For this review, take the finished solid that the model builds, in its own axes (mm). A direction names the side the tool comes from. Give positions to 0.01 mm unless a question says otherwise; leave off trailing zeros. Loops run counter-clockwise (first coordinate to the right, second up) from the corner with the lowest first, then second, coordinate; pieces in that order, holes last. Notation, with made-up numbers: (73, 65.25) - (91, 65.25) arc R33 ccw to (91, 99.25) - close; hole circle Ø6 at (88, -34.75). An arc over 180 degrees is marked (long way). Answer in a Markdown table with one row per item.
```python
from build123d import *

# Parameters (mm, degrees)
F0_W     = 136.525
F0_H     = 241.3
F1_DEPTH = 25.4
F3_DEPTH = 25.4


with BuildPart() as f1:
    # F0 (on Front) → F1 (new body)
    with BuildSketch(Plane.XZ):
        Rectangle(F0_W, F0_H)
    extrude(amount=F1_DEPTH)

    # F2 (on face) → F3 (join)
    with BuildSketch(Plane.XZ.offset(25.4)):
        with BuildLine():
            ThreePointArc((77.6254340957, 53.8129340957), (71.9080698474, 61.2266782869), (68.2625, 69.85))
            Line((68.2625, 69.85), (68.2625, -6.35))
            ThreePointArc((68.2625, -6.35), (71.9080698474, 2.2733217131), (77.6254340957, 9.6870659043))
            ThreePointArc((77.6254340957, 9.6870659043), (82.7346936877, 13.9409024845), (88.5302033496, 17.1984670639))
            ThreePointArc((88.5302033496, 17.1984670639), (92.3418278085, 24.0349565831), (93.6625, 31.75))
            ThreePointArc((93.6625, 31.75), (92.3418278085, 39.4650434169), (88.5302033496, 46.3015329361))
            ThreePointArc((88.5302033496, 46.3015329361), (82.7346936877, 49.5590975155), (77.6254340957, 53.8129340957))
        make_face()
        with BuildLine():
            ThreePointArc((88.5302033496, 46.3015329361), (83.6252121519, 50.8519186766), (77.6254340957, 53.8129340957))
            ThreePointArc((77.6254340957, 53.8129340957), (82.7346936877, 49.5590975155), (88.5302033496, 46.3015329361))
        make_face()
        with BuildLine():
            ThreePointArc((88.5302033496, 17.1984670639), (82.7346936877, 13.9409024845), (77.6254340957, 9.6870659043))
            ThreePointArc((77.6254340957, 9.6870659043), (83.6252121519, 12.6480813234), (88.5302033496, 17.1984670639))
        make_face()
    extrude(amount=-F3_DEPTH)

    # F4: F1 across plane


with BuildPart() as f1_1:
    add(f1.part)
    add(f1.part.mirror(Plane.YZ))


solid = f1_1.part
```
1. Wall thickness on line 1 (X direction, y = -1.5, z = 70); line 2 (X direction, y = -7.5, z = 33); line 3 (Z direction, x = 71.5, y = -16.75): over which ranges is each line inside the solid? List them lowest first. Write a range as [from, to].
Values:
| item | result |
|---|---|
| line 1 | x = [-68.26, 68.26] |
| line 2 | x = [-93.63, 93.63] |
| line 3 | z = [1.56, 61.94] |
2. Clearance check with flat-ended pins moving along their axes: pin 1 (4 mm diameter, centred on y = -18.5, z = -6, fed in from +X); pin 2 (12.5 mm diameter, centred on y = -18, z = -74.5, fed in from +X); pin 3 (12.5 mm diameter, centred on y = -15, z = -78, fed in from -X). State where each tip first meets the part, or that it passes through.
Values:
| item | result |
|---|---|
| pin 1 | stops at x = 69 |
| pin 2 | stops at x = 68.26 |
| pin 3 | stops at x = -68.26 |
3. For faces 1 (the face through (68.262, -13, 95)), 2 (the face through (-68.262, -13, 95)), 3 (the face through (-68.262, -13, -64)), list the 3-axis set-ups (+Z, -Z, +X, -X, +Y, -Y) from which the entire face can be reached by the end or side of a thin tool; tool diameter is ignored.
Values:
| item | result |
|---|---|
| face 1 | +Z, +X, +Y, -Y |
| face 2 | +Z, -X, +Y, -Y |
| face 3 | -Z, -X, +Y, -Y |
4. We need section A-A, the plane y = -7.75. Give the boundary of the cut face in (x, z), and give its area (3 significant figures).
Values:
| item | result |
|---|---|
| outline | (-77.63, 9.69) arc R36.54 cw to (-68.26, -6.35) - (-68.26, -120.65) - (68.26, -120.65) - (68.26, -6.35) arc R36.54 cw to (77.63, 9.69) arc R23.2 ccw to (77.63, 53.81) arc R36.54 cw to (68.26, 69.85) - (68.26, 120.65) - (-68.26, 120.65) - (-68.26, 69.85) arc R36.54 cw to (-77.63, 53.81) arc R23.2 ccw to start |
| area | 35,000 mm^2 |
5. We need section B-B, the plane z = 94. Give the boundary of the cut face in (x, y), and give its area (3 significant figures).
Values:
| item | result |
|---|---|
| outline | (-68.26, -25.4) - (68.26, -25.4) - (68.26, 0) - (-68.26, 0) - close |
| area | 3,470 mm^2 |
6. We need section C-C, the plane x = -72.5. Give the boundary of the cut face in (y, z).
Values:
| item | result |
|---|---|
| outline | (-25.4, 3.25) - (0, 3.25) - (0, 60.25) - (-25.4, 60.25) - close |
